Read the model definition and answer for the solid it produces. Units are mm, in the model's axes. A direction names the side the tool comes from. Give positions to 0.01 mm unless a question says otherwise; leave off trailing zeros. Loops run counter-clockwise (first coordinate to the right, second up) from the corner with the lowest first, then second, coordinate; pieces in that order, holes last. Notation, with made-up numbers: (20, -17.75) -> (56, -17.75) arc R13 cw to (56, -4.75) -> close; hole circle Ø5 at (-18.5, 53). An arc over 180 degrees is marked (long way). One line per item, written item: value. Start each with the question number.
Autodesk Inventor part; units mm, degrees
ref_plane "YZ Plane" through (0, 0, 0) normal (1, 0, 0) x (0, 1, 0)
ref_plane "XZ Plane" through (0, 0, 0) normal (0, 1, 0) x (-1, 0, 0)
ref_plane "XY Plane" through (0, 0, 0) normal (0, 0, 1) x (1, 0, 0)
sketch "Sketch1" plane through (0, 0, 0) normal (1, 0, 0) x (0, 1, 0)
  circle A0 centre (0, 0) radius 50
  dimension "d0" = 100
extrude "Extrusion1" add sketch "Sketch1" along normal blind 10
sketch "Sketch2" plane through (10, 0, 0) normal (1, 0, 0) x (0, 0, -1)
  circle A0 centre (0, 0) radius 50
hole "Hole1" at (10, 0, 0) direction (-1, 0, 0) diameter 12 depth 10
fillet "Fillet1" radius 2 2 edges at (0, -50, 0) (10, -50, 0)
sketch "Sketch4" plane through (10, 0, 0) normal (1, 0, 0) x (0, 0, -1)
  circle A0 centre (0, 0) radius 15
  dimension "d18" = 30
extrude "Extrusion3" cut sketch "Sketch4" against normal blind 3
sketch "Sketch5" plane through (7, 0, 0) normal (1, 0, 0) x (0, 0, -1)
  circle A0 centre (0, 0) radius 6
  line L0 (-6, 0) -> (-6, 2)
  line L1 (-6, 2) -> (-8, 2)
  line L2 (-8, 2) -> (-8, -2)
  line L3 (-8, -2) -> (-6, -2)
  line L4 (-6, -2) -> (-6, 0)
  line L5 (-6, -2) -> (-4.5, -2)
  line L6 (-4.5, -2) -> (-4.5, 2)
  line L7 (-4.5, 2) -> (-6, 2)
  point P0 (-7, -2)
  dimension "d21" = 2
  dimension "d22" = 4
  dimension "d23" = 2
  dimension "d24" = 1.5
  dimension "d25" = 4
extrude "Extrusion4" cut sketch "Sketch5" against normal blind 7 contours L7 L6 L5 A0 | A0 L0 L7 | L5 L4 A0 | L4 L3 L2 L1 L0 picked at (-5, 0)
properties part number "P203" material "Aluminum 6061"
Item 1: Consider L1, parallel to Z at x = 3, y = 0; L2, parallel to Y at x = 8.5, z = 1.5; L3, parallel to X at y = -10.5, z = 8.5. Determine where each line is inside the solid, lowest interval first. Write a range as [from, to].
Item 2: Flat-ended cylindrical pins translate along their axes: pin 1 (6 mm diameter, centred on x = 5, y = -10.5, fed in from +Z); pin 2 (2 mm diameter, centred on x = 2, z = 13.5, fed in from -Y); pin 3 (19 mm diameter, centred on y = 0, z = 0, fed in from +X). Find the tip coordinate at first contact, or state that the pin passes through.
Item 3: For faces 4 (the flat face through (4, 0, 8)), 5 (the flat face through (10, -11, 11)), 6 (the cylindrical face through (8.521, 0.66, 14.985)), determine the directions among +Z, -Z, +X, -X, +Y, -Y from which every point of the face is accessible in a straight line to the end or side of a thin tool.
Item 4: Determine the mould class of faces 1 (the flat face through (0, 10, 1)), 2 (the cylindrical face through (4.96, 47.69, -15.02)), 3 (the flat face through (7, 0.2, -6.5)) for opening direction Z: pulls with the +Z half, pulls with the -Z half, needs draft (parallel to the pull), parting line crosses it, or undercut.
Item 5: Section A-A, the plane y = 0 is taken. Determine the outline of the cut face in (x, z), plus the area to 3 significant figures.
Item 6: Section B-B, the plane z = 0 is taken. Determine the outline of the cut face in (x, y).
Computed values:
1. L1: [-50, -6], [8, 50]
1. L2: [-49.91, -14.92], [14.92, 49.91]
1. L3: [0, 7]
2. pin 1: z = 49.43
2. pin 2: y = -48.41
2. pin 3: x = 7
3. face 4: +X, -X
3. face 5: +Z, -Z, +X, +Y, -Y
3. face 6: +X
4. face 1: needs draft
4. face 2: parting line crosses it
4. face 3: undercut
5. outline: (0, -48) arc R2 ccw to (2, -50) -> (8, -50) arc R2 ccw to (10, -48) -> (10, -15) -> (7, -15) -> (7, -6) -> (0, -6) -> close; (0, 8) -> (7, 8) -> (7, 15) -> (10, 15) -> (10, 48) arc R2 ccw to (8, 50) -> (2, 50) arc R2 ccw to (0, 48) -> close
5. area: 809 mm²
6. outline: (0, -48) arc R2 ccw to (2, -50) -> (8, -50) arc R2 ccw to (10, -48) -> (10, -15) -> (7, -15) -> (7, -6) -> (0, -6) -> close; (0, 6) -> (7, 6) -> (7, 15) -> (10, 15) -> (10, 48) arc R2 ccw to (8, 50) -> (2, 50) arc R2 ccw to (0, 48) -> close
